```python
from build123d import *

# Parameters (mm, degrees)
F2_R = 1.016
F3_W = 0.635
F3_H = 0.635
F5_R = 1.016


with BuildPart() as f1:
    # F0 (on Front) → F1 (revolve)
    with BuildSketch(Plane.XZ):
        Polygon((0, 38.1), (0, 0), (11.43, 0), (11.43, 1.27), (3.175, 4.274574), (3.175, 38.1), align=None)
    revolve(axis=Axis((0, 0, 19.05), (0, 0, -1)))

    # F2
    f2_edges = [f1.edges().sort_by_distance(p)[0] for p in [
        (-11.43, 0, 1.27),
        (-3.175, 0, 4.274574),
    ]]
    fillet(f2_edges, radius=F2_R)

    # F3 (on Front) → F4 (revolve, cut)
    with BuildSketch(Plane.XZ):
        with Locations((2.8575, 35.2425)):
            Rectangle(F3_W, F3_H)
    revolve(axis=Axis((0, 0, 4.274574), (0, 0, 1)), mode=Mode.SUBTRACT)

    # F5
    f5_edges = [f1.edges().sort_by_distance(p)[0] for p in [
        (-3.175, 0, 38.1),
    ]]
    fillet(f5_edges, radius=F5_R)


solid = f1.part
```
Check sheet for the modelled part. Datum: model origin and axes. Units: mm. A direction names the side the tool comes from. Give positions to 0.01 mm unless a question says otherwise; leave off trailing zeros. Order: outer loops, then holes, each group sorted by start corner. A loop starts at its lowest first (then second) coordinate and runs counter-clockwise, first axis right, second up. Notation, with made-up numbers: M 41,35.5 L 60,35.5 A16 ccw 60,49.5 Z; hole C 78.25,-21.75 d1. An arc over 180 degrees is marked long. Answer in a Markdown table with one row per item.
1) Cross-section at A-A, the plane z = 5.5. Enter the section's corners in (x, y) (3 decimals), plus the area to 3 significant figures.
Filled sheet:
| item | result |
|---|---|
| outline | C 0,0 d6.35 |
| area | 31.7 mm2 |
2) Thickness scan on L1, parallel to Z at x = -3, y = -0.5 (3 decimals); L2, parallel to X at y = 0.5, z = 12; L3, parallel to Y at x = 2.5, z = 20. Record the ranges inside material, lowest first. Write a range as [from, to].
Filled sheet:
| item | result |
|---|---|
| L1 | z = [0, 34.925], [35.56, 37.588] |
| L2 | x = [-3.14, 3.14] |
| L3 | y = [-1.96, 1.96] |
3) Release check for a two-part mould opening along Z. For faces 4 (the flat face through (0, 0, 0)), 5 (the cylindrical face through (-2.34, -2.146, 20.165)), 6 (the flat face through (0, 0, 38.1)), 7 (the flat face through (0, 3, 34.925)) record: +Z half, -Z half, draft (parallel to the pull), parting line (faces both ways), or undercut.
Filled sheet:
| item | result |
|---|---|
| face 4 | -Z half |
| face 5 | draft |
| face 6 | +Z half |
| face 7 | undercut |
4) Gauge pin test, flat ends, axial feed: P1, Ø4, axis at x = 1, z = 30.5, coming from the -Y side (3 decimals); P2, Ø3, axis at x = -1, y = 0.5, coming from the -Z side; P3, Ø1.5, axis at x = 3.5, y = -2.5, coming from the +Z side; P4, Ø3, axis at x = -4, y = 6.5, coming from the +Z side. Record the tip position at first contact, or that the pin passes through.
Filled sheet:
| item | result |
|---|---|
| P1 | stops at y = -3.175 |
| P2 | stops at z = 0 |
| P3 | stops at z = 4.2 |
| P4 | stops at z = 3.2 |
5) Access from +Z, -Z, +X, -X, +Y, -Y to the whole of each face (thin tool, end or side, straight path). Record for faces 1 (the cylindrical face through (-0.69, 3.1, 36.33)), 2 (the flat face through (0, 3, 35.56)), 3 (the cylindrical face through (10.902, -3.433, 0.283)).
Filled sheet:
| item | result |
|---|---|
| face 1 | +Z |
| face 2 | none |
| face 3 | +Z, -Z |
